Study the drawing (mm; zero at the part's minimum x, y, z) and answer. A direction names the side the tool comes from. Coordinates: 2 decimals unless noted, no trailing zeros. Order: outer loops, then holes, each group sorted by start corner. A loop starts at its lowest first (then second) coordinate and runs counter-clockwise, first axis right, second up.
1. The part is cut by section A-A, the plane x = 44.3. Give the vertices of the cut face in (y, z), then the cut area to 3 significant figures.
2. Find the intervals of material crossed by probe 1 along X at (y, z) = (27.9, 19.25); probe 2 along Z at (x, y) = (32, 11.5); probe 3 along X at (y, z) = (28.5, 20), in increasing order.
3. The part is cut by section B-B, the plane y = 27.9. Give the vertices of the cut face in (x, z).
4. The part is cut by section C-C, the plane z = 21. Give the vertices of the cut face in (x, y), then the cut area to 3 significant figures.
5. A tool of negligible diameter and unlimited length cuts with its end or side. For the marked faces 4, 5 and 6, from which of +Z, -Z, +X, -X, +Y, -Y can it reach the whole face along a straight path? Write none if from no direction.
6. Determine the mould class of the marked faces 1, 2 and 3 for opening direction Y: +Y half, -Y half, draft (parallel to the pull), parting line (faces both ways), or undercut.
7. The part is cut by section D-D, the plane x = 56. Give the vertices of the cut face in (y, z).
8. Flat-ended cylindrical pins translate along their axes: pin 1 Ø2.5 at (y, z) = (11, 12) entering from +X; pin 2 Ø2.5 at (y, z) = (26.5, 2.5) entering from +X; pin 3 Ø4.5 at (x, y) = (59.9, 27.9) entering from -Z; pin 4 Ø2 at (x, z) = (51, 15) entering from +Y. Find the tip coordinate at first contact, or state that the pin passes through.
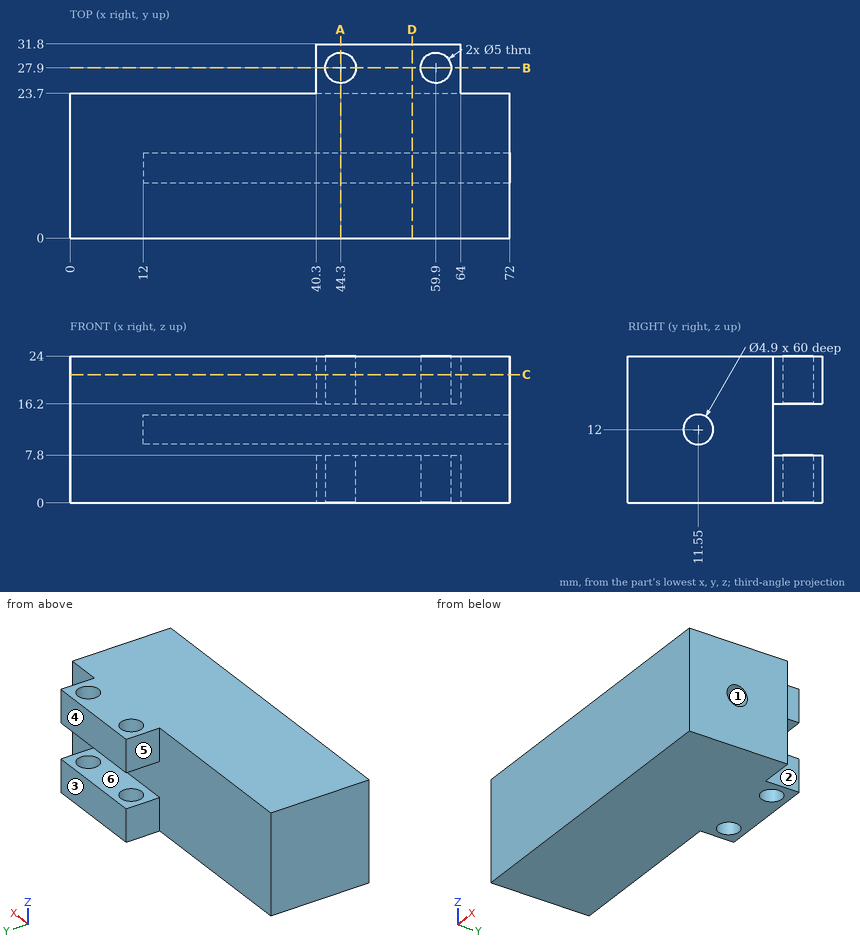
Geometry says:
1. outline: (0, 0) - (25.4, 0) - (25.4, 7.8) - (23.7, 7.8) - (23.7, 16.2) - (25.4, 16.2) - (25.4, 24) - (0, 24) - close; (30.4, 0) - (31.8, 0) - (31.8, 7.8) - (30.4, 7.8) - close; (30.4, 16.2) - (31.8, 16.2) - (31.8, 24) - (30.4, 24) - close; hole circle Ø4.9 at (11.55, 12)
1. area: 598 mm2
2. probe 1: x = 40.3 to 41.8, 46.8 to 57.4, 62.4 to 64
2. probe 2: z = 0 to 9.55, 14.45 to 24
2. probe 3: x = 40.3 to 41.87, 46.73 to 57.47, 62.33 to 64
3. outline: (40.3, 0) - (41.8, 0) - (41.8, 7.8) - (40.3, 7.8) - close; (40.3, 16.2) - (41.8, 16.2) - (41.8, 24) - (40.3, 24) - close; (46.8, 0) - (57.4, 0) - (57.4, 7.8) - (46.8, 7.8) - close; (46.8, 16.2) - (57.4, 16.2) - (57.4, 24) - (46.8, 24) - close; (62.4, 0) - (64, 0) - (64, 7.8) - (62.4, 7.8) - close; (62.4, 16.2) - (64, 16.2) - (64, 24) - (62.4, 24) - close
4. outline: (0, 0) - (72, 0) - (72, 23.7) - (64, 23.7) - (64, 31.8) - (40.3, 31.8) - (40.3, 23.7) - (0, 23.7) - close; hole circle Ø5 at (44.3, 27.9); hole circle Ø5 at (59.9, 27.9)
4. area: 1,860 mm2
5. face 4: +Z, -Z, +X, -X, +Y
5. face 5: +Z, -Z, -X, +Y
5. face 6: +X, -X, +Y
6. face 1: undercut
6. face 2: draft
6. face 3: +Y half
7. outline: (0, 0) - (31.8, 0) - (31.8, 7.8) - (23.7, 7.8) - (23.7, 16.2) - (31.8, 16.2) - (31.8, 24) - (0, 24) - close; hole circle Ø4.9 at (11.55, 12)
8. pin 1: stops at x = 12
8. pin 2: stops at x = 64
8. pin 3: passes through
8. pin 4: stops at y = 23.7
